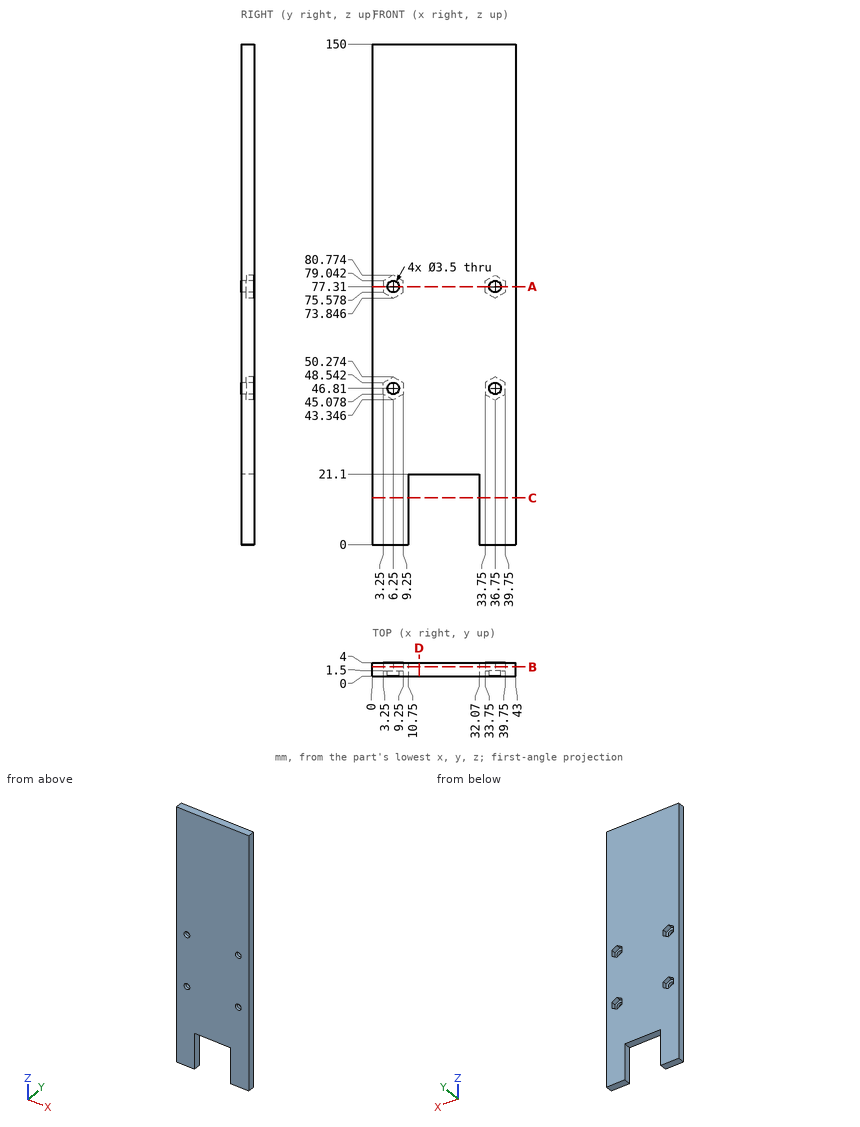
Check sheet for the drawn part. Datum: minimum x, y, z corner. Units: mm. Round coordinates to 2 decimals unless told otherwise and drop trailing zeros. Order: outer loops, then holes, each group sorted by start corner. A loop starts at its lowest first (then second) coordinate and runs counter-clockwise, first axis right, second up. Notation, with made-up numbers: M -5.5,23.5 L 18.5,23.5 A24 ccw 18.5,46.5 Z; hole C 11.5,58 d9. An arc over 180 degrees is marked long. Answer in a Markdown table with one row per item.
(1) Section check C-C on z = 14. Record the boundary of the cut face in (x, y).
Findings:
| item | result |
|---|---|
| outline | M 0,0 L 10.75,0 L 10.75,4 L 0,4 Z; M 32.07,0 L 43,0 L 43,4 L 32.07,4 Z |
(2) Gauge pin test, flat ends, axial feed: pin 1 (4 mm diameter, centred on x = 36.75, z = 77.31, fed in from +Y); pin 2 (1.2 mm diameter, centred on x = 25.5, y = 1.5, fed in from -Z); pin 3 (3 mm diameter, centred on x = 6.25, z = 77.31, fed in from -Y). Record the tip position at first contact, or that the pin passes through.
Findings:
| item | result |
|---|---|
| pin 1 | stops at y = 1.5 |
| pin 2 | stops at z = 21.1 |
| pin 3 | passes through |
(3) Material ranges on line 1 along X through (y, z) = (1.2, 77.31); line 2 along Z through (x, y) = (7.5, 0.3) (1 decimal); line 3 along Z through (x, y) = (35, 3.75), recorded low to high. Write a range as from..to.
Findings:
| item | result |
|---|---|
| line 1 | x = 0..4.5, 8..35, 38.5..43 |
| line 2 | z = 0..45.6, 48..76.1, 78.5..150 |
| line 3 | z = 0..44.36, 49.26..74.86, 79.76..150 |
(4) Section check B-B on y = 2.7. Give the number of separate pieces and of enclosed holes in the cut face, plus the area to 3 significant figures.
Findings:
| item | result |
|---|---|
| separate pieces | 1 |
| enclosed holes | 4 |
| area | 5,880 mm^2 |
(5) Section check A-A on z = 77.31. Record the boundary of the cut face in (x, y).
Findings:
| item | result |
|---|---|
| outline | M 0,0 L 4.5,0 L 4.5,1.5 L 3.25,1.5 L 3.25,4 L 0,4 Z; M 8,0 L 35,0 L 35,1.5 L 33.75,1.5 L 33.75,4 L 9.25,4 L 9.25,1.5 L 8,1.5 Z; M 38.5,0 L 43,0 L 43,4 L 39.75,4 L 39.75,1.5 L 38.5,1.5 Z |
(6) Section check D-D on x = 14. Record the boundary of the cut face in (y, z).
Findings:
| item | result |
|---|---|
| outline | M 0,21.1 L 4,21.1 L 4,150 L 0,150 Z |
